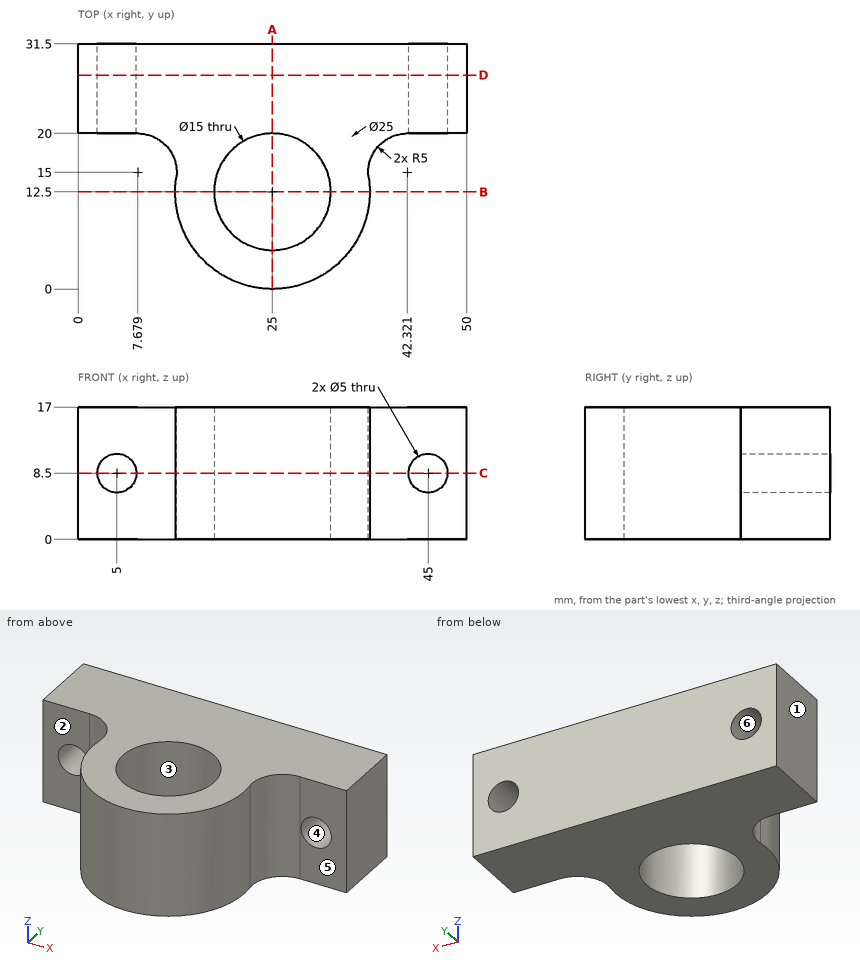
Geometry: see drawing. Coordinates: mm, zero at the bounding-box minimum. A direction names the side the tool comes from. Round coordinates to 2 decimals unless told otherwise and drop trailing zeros. Loops run counter-clockwise (first coordinate to the right, second up) from the corner with the lowest first, then second, coordinate; pieces in that order, holes last.
(1) Pull-direction query (X, two-part tool) for the marked faces 1, 2, 3 and 4; classes: +X half, -X half, draft (parallel to the pull), parting line (faces both ways), or undercut.
From the geometry:
face 1: -X half
face 2: draft
face 3: undercut
face 4: undercut
(2) Section query A-A (x = 25). Output: boundary loops of the cut face in (y, z).
From the geometry:
outline: (0, 0) - (5, 0) - (5, 17) - (0, 17) - close; (20, 0) - (31.5, 0) - (31.5, 17) - (20, 17) - close
(3) Access query for the marked faces 5 and 6. Directions: +Z, -Z, +X, -X, +Y, -Y. A direction counts if a zero-diameter tool reaches every point of the face in a straight line with its end or side. Return the directions, or none.
From the geometry:
face 5: +Z, -Z, +X, -Y
face 6: +Y, -Y
(4) Material intervals for probe 1 along X at (y, z) = (23, 8.5); probe 2 along Y at (x, z) = (25, 4.75); probe 3 along Z at (x, y) = (5, 25), sorted ascending.
From the geometry:
probe 1: x = 0 to 2.5, 7.5 to 42.5, 47.5 to 50
probe 2: y = 0 to 5, 20 to 31.5
probe 3: z = 0 to 6, 11 to 17
(5) Section query C-C (z = 8.5). Give the number of separate pieces and of enclosed holes in the cut face, and give its area (3 significant figures).
From the geometry:
separate pieces: 3
enclosed holes: 1
area: 725 mm2
(6) Contact query for flat-ended pins moving along their axis: pin 1 Ø2 at (x, y) = (32.5, 7) entering from -Z; pin 2 Ø6.5 at (x, z) = (5, 8.5) entering from -Y; pin 3 Ø5 at (y, z) = (9, 4.5) entering from +X; pin 4 Ø4 at (x, z) = (13.5, 5) entering from -Y (1 decimal). Output: stop coordinate, or through.
From the geometry:
pin 1: stops at z = 0
pin 2: stops at y = 19.97
pin 3: stops at x = 37.46
pin 4: stops at y = 4.4
(7) Section query B-B (y = 12.5). Output: boundary loops of the cut face in (x, z).
From the geometry:
outline: (12.5, 0) - (17.5, 0) - (17.5, 17) - (12.5, 17) - close; (32.5, 0) - (37.5, 0) - (37.5, 17) - (32.5, 17) - close
(8) Section query D-D (y = 27.5). Output: boundary loops of the cut face in (x, z), and give its area (3 significant figures).
From the geometry:
outline: (0, 0) - (50, 0) - (50, 17) - (0, 17) - close; hole circle Ø5 at (5, 8.5); hole circle Ø5 at (45, 8.5)
area: 811 mm2
